Here's the drawing with two shaded views (mm, measured from the low corner). I have some questions. Coordinates: 2 decimals unless noted, no trailing zeros. Write each loop counter-clockwise with the first axis right and the second up, starting at its lowest first coordinate (ties: lowest second). Pieces come first, ordered by that corner, then holes. Notation, with made-up numbers: (-7.75, 29.5) -> (32.25, 29.5) arc R32 cw to (32.25, 65.5) -> close; hole circle Ø2 at (-38.75, -15). An arc over 180 degrees is marked (long way). Put each result on its own line as item: value. Start each with the question number.
Item 1: For pin 1 (2.5 mm diameter, centred on x = 4.5, y = 22.5, fed in from -Z), with a flat end and sliding along its axis, tell me the tip position at first contact or that it passes through.
Item 2: I want a section at B-B, the plane z = 2. State how many separate pieces and enclosed holes the cut face has, then the cut area to 3 significant figures.
Item 3: I want a section at D-D, the plane y = 22. List the corners of the cut face in (x, z) for me, then the cut area to 3 significant figures.
Item 4: I want a section at C-C, the plane y = 13.5. List the corners of the cut face in (x, z) for me.
Item 5: I want a section at A-A, the plane x = 13.5. List the corners of the cut face in (y, z) for me.
Item 6: I need wall thicknesses on line 1 (Y direction, x = 4.5, z = 0.7); line 2 (X direction, y = 40, z = 1.85); line 3 (X direction, y = 42.5, z = 0.3). Which ranges of each line are inside material? Lowest first, please. Write a range as [from, to].
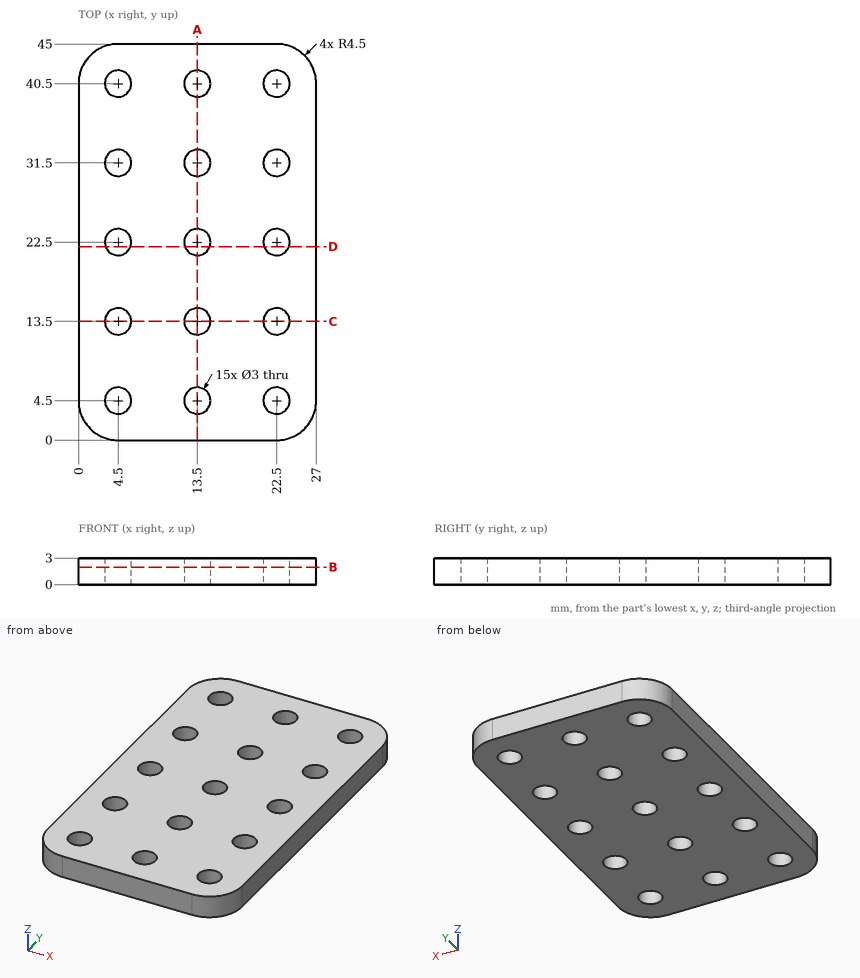
Calculated:
1. pin 1: passes through
2. separate pieces: 1
2. enclosed holes: 15
2. area: 1,090 mm2
3. outline: (0, 0) -> (3.09, 0) -> (3.09, 3) -> (0, 3) -> close; (5.91, 0) -> (12.09, 0) -> (12.09, 3) -> (5.91, 3) -> close; (14.91, 0) -> (21.09, 0) -> (21.09, 3) -> (14.91, 3) -> close; (23.91, 0) -> (27, 0) -> (27, 3) -> (23.91, 3) -> close
3. area: 55.5 mm2
4. outline: (0, 0) -> (3, 0) -> (3, 3) -> (0, 3) -> close; (6, 0) -> (12, 0) -> (12, 3) -> (6, 3) -> close; (15, 0) -> (21, 0) -> (21, 3) -> (15, 3) -> close; (24, 0) -> (27, 0) -> (27, 3) -> (24, 3) -> close
5. outline: (0, 0) -> (3, 0) -> (3, 3) -> (0, 3) -> close; (6, 0) -> (12, 0) -> (12, 3) -> (6, 3) -> close; (15, 0) -> (21, 0) -> (21, 3) -> (15, 3) -> close; (24, 0) -> (30, 0) -> (30, 3) -> (24, 3) -> close; (33, 0) -> (39, 0) -> (39, 3) -> (33, 3) -> close; (42, 0) -> (45, 0) -> (45, 3) -> (42, 3) -> close
6. line 1: y = [0, 3], [6, 12], [15, 21], [24, 30], [33, 39], [42, 45]
6. line 2: x = [0, 3.09], [5.91, 12.09], [14.91, 21.09], [23.91, 27]
6. line 3: x = [0.47, 26.53]
